The drawing under review shows one solid part. Ordinate dimensions are in mm from its lowest x, y, z. A direction names the side the tool comes from. Give positions to 0.01 mm unless a question says otherwise; leave off trailing zeros. Loops run counter-clockwise (first coordinate to the right, second up) from the corner with the lowest first, then second, coordinate; pieces in that order, holes last. Notation, with made-up numbers: (20, -7.75) - (24, -7.75) arc R30 ccw to (24, 27.25) - close; hole circle Ø6 at (-21.75, 30). An arc over 180 degrees is marked (long way). Put each result on its own line as item: value. Start each with the question number.
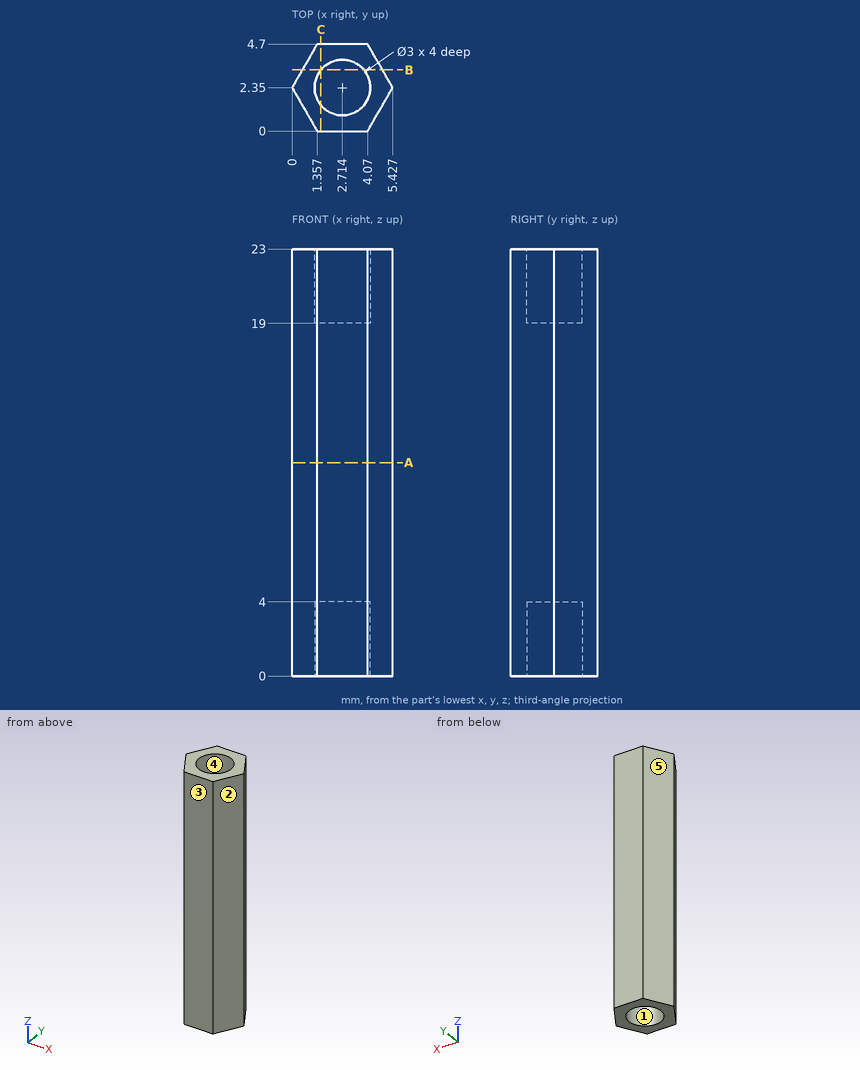
Item 1: Machinability: for the marked faces 4 and 5, which of the approach directions +Z, -Z, +X, -X, +Y, -Y give a long, thin tool a straight path to every point of the face, cutting with its end or side? Answer none if there is none.
Item 2: Consider section C-C (x = 1.55). State the section outline as (y, z) points.
Item 3: Mouldability with a two-part tool opening along X and no side actions: class the marked faces 1, 2 and 3 as pulls with the +X half, pulls with the -X half, needs draft (parallel to the pull), parting line crosses it, or undercut.
Item 4: Consider section B-B (y = 3.3). State the section outline as (x, z) points (1 decimal).
Item 5: Consider section A-A (z = 11.5). State the section outline as (x, y) points.
Item 6: For P1, Ø1.8, axis at x = 2.71, y = 2.35, coming from the +Z side; P2, Ø1, axis at y = 0.5, z = 7, coming from the -X side; P3, Ø2, axis at y = 2.5, z = 5, coming from the -X side, all flat-tipped, find the tip position at first contact; note any pin that passes through.
Item 7: For L1, parallel to Z at x = 2.55, y = 3.75; L2, parallel to X at y = 3.6, z = 2.5 (1 decimal); L3, parallel to Y at x = 0.95, z = 12.5 (1 decimal), list the stretches that pass through material, from the lowest coordinate up. Write a range as from..to.
Geometry says:
1. face 4: +Z
1. face 5: +Z, -Z, -X, +Y
2. outline: (0, 0) - (1.4, 0) - (1.4, 4) - (3.3, 4) - (3.3, 0) - (4.7, 0) - (4.7, 23) - (3.3, 23) - (3.3, 19) - (1.4, 19) - (1.4, 23) - (0, 23) - close
3. face 1: undercut
3. face 2: pulls with the +X half
3. face 3: needs draft
4. outline: (0.5, 0) - (1.6, 0) - (1.6, 4) - (3.9, 4) - (3.9, 0) - (4.9, 0) - (4.9, 23) - (3.9, 23) - (3.9, 19) - (1.6, 19) - (1.6, 23) - (0.5, 23) - close
5. outline: (0, 2.35) - (1.36, 0) - (4.07, 0) - (5.43, 2.35) - (4.07, 4.7) - (1.36, 4.7) - close
6. P1: stops at z = 19
6. P2: stops at x = 0.78
6. P3: stops at x = 0
7. L1: z = 4..19
7. L2: x = 0.7..1.9, 3.5..4.7
7. L3: y = 0.7..4
